The listing builds one solid part. Answer for the finished solid, in the listing's coordinates (mm). A direction names the side the tool comes from. Round coordinates to 2 decimals unless told otherwise and drop trailing zeros. Write each loop counter-clockwise with the first axis right and the second up, starting at its lowest first coordinate (ties: lowest second). Pieces come first, ordered by that corner, then holes.
from build123d import *

# Parameters (mm, degrees)
F1_DEPTH  = 210
F2_DEPTH  = 210
F3_DEPTH  = 60
F5_D      = 15
F5_DEPTH  = 40
F5_TIP    = 4.5064546427
F7_DEPTH  = 20
F9_DEPTH  = 20
F10_W     = 10
F10_H     = 20
F11_DEPTH = 210
F12_D     = 10
F12_DEPTH = 40
F12_TIP   = 3.0043030951
F13_R     = 7
F14_DEPTH = 50
F15_R     = 7
F16_DEPTH = 50
F18_D     = 15
F18_DEPTH = 220
F18_TIP   = 4.5064546427
F19_W     = 60
F19_H     = 50
F20_DEPTH = 60
F21_W     = 9.6634474397
F21_H     = 30
F21_W_2   = 10
F22_DEPTH = 20
F23_DEPTH = 25
F24_DEPTH = 31
F25_DEPTH = 37
F26_DEPTH = 45
F27_DEPTH = 120
F28_DEPTH = 105
F29_DEPTH = 200


with BuildPart() as f1:
    # F0 (on Front) → F1 (new body)
    with BuildSketch(Plane.XZ):
        with BuildLine():
            Line((-190, 0), (-210, 0))
            ThreePointArc((-210, 0), (-148.4924240492, -148.4924240492), (0, -210))
            Line((0, -210), (0, -190))
            ThreePointArc((0, -190), (-134.3502884254, -134.3502884254), (-190, 0))
        make_face()
    extrude(amount=F1_DEPTH)

    # F2 (add): a face of the model
    f2_faces = [f1.faces().sort_by_distance(p)[0] for p in [
        (-200, -105, 0),
    ]]
    extrude(f2_faces, amount=-F2_DEPTH)

    # F3 (add): a face of the model
    f3_faces = [f1.faces().sort_by_distance(p)[0] for p in [
        (0, -105, -200),
    ]]
    extrude(f3_faces, amount=-F3_DEPTH)

    # F5
    with Locations(Plane(origin=(0, 0, -210), x_dir=(1, 0, 0), z_dir=(0, 0, -1))):
        with Locations((-30, 157.5), (-30, 52.5)):
            Hole(F5_D / 2, depth=F5_DEPTH)
            with Locations((0, 0, -(F5_DEPTH + F5_TIP / 2))):  # 118° drill point
                Cone(0, F5_D / 2, F5_TIP, mode=Mode.SUBTRACT)

    # F6 (on face) → F7 (join)
    with BuildSketch(Plane.XZ.offset(210)):
        with BuildLine():
            ThreePointArc((0, -170), (-120.2081528017, -120.2081528017), (-170, 0))
            Line((-170, 0), (-190, 0))
            ThreePointArc((-190, 0), (-134.3502884254, -134.3502884254), (0, -190))
            Line((0, -190), (0, -170))
        make_face()
    extrude(amount=-F7_DEPTH)

    # F8 (on face) → F9 (join)
    with BuildSketch(Plane(origin=(0, 0, 0), x_dir=(-1, 0, 0), z_dir=(0, 1, 0))):
        with BuildLine():
            Line((190, 0), (170, 0))
            ThreePointArc((170, 0), (120.2081528017, -120.2081528017), (0, -170))
            Line((0, -170), (0, -190))
            ThreePointArc((0, -190), (134.3502884254, -134.3502884254), (190, 0))
        make_face()
    extrude(amount=-F9_DEPTH)

    # F10 (on face) → F11 (join)
    with BuildSketch(Plane.XZ.offset(210)):
        with Locations((-35, -200)):
            Rectangle(F10_W, F10_H)
        with Locations((-25, -200)):
            Rectangle(F10_W, F10_H)
    extrude(amount=-F11_DEPTH)

    # F12
    with Locations(Plane(origin=(0, 0, -210), x_dir=(1, 0, 0), z_dir=(0, 0, -1))):
        with Locations((-30, 157.5), (-30, 52.5)):
            Hole(F12_D / 2, depth=F12_DEPTH)
            with Locations((0, 0, -(F12_DEPTH + F12_TIP / 2))):  # 118° drill point
                Cone(0, F12_D / 2, F12_TIP, mode=Mode.SUBTRACT)

    # F13 (on face) → F14 (cut)
    with BuildSketch(Plane.YZ):
        with Locations((-140, -200)):
            Circle(F13_R)
        with Locations((-105, -200)):
            Circle(F13_R)
        with Locations((-70, -200)):
            Circle(F13_R)
    extrude(amount=-F14_DEPTH, mode=Mode.SUBTRACT)

    # F15 (on face) → F16 (cut)
    with BuildSketch(Plane.XY):
        with Locations((-200, -35)):
            Circle(F15_R)
        with Locations((-200, -70)):
            Circle(F15_R)
        with Locations((-200, -105)):
            Circle(F15_R)
        with Locations((-200, -140)):
            Circle(F15_R)
        with Locations((-200, -175)):
            Circle(F15_R)
    extrude(amount=-F16_DEPTH, mode=Mode.SUBTRACT)

    # F18
    with Locations(Plane.XZ.offset(210)):
        with Locations((-183.5259069949, -49.1756185695), (-164.544826719, -95), (-134.3502884254, -134.3502884254), (-49.1756185695, -183.5259069949)):
            Hole(F18_D / 2, depth=F18_DEPTH)
            with Locations((0, 0, -(F18_DEPTH + F18_TIP / 2))):  # 118° drill point
                Cone(0, F18_D / 2, F18_TIP, mode=Mode.SUBTRACT)

    # F19 (on face) → F20 (cut)
    with BuildSketch(Plane(origin=(0, 0, -210), x_dir=(1, 0, 0), z_dir=(0, 0, -1))):
        with Locations((-100, 105)):
            Rectangle(F19_W, F19_H)
    extrude(amount=-F20_DEPTH, mode=Mode.SUBTRACT)

    # F21 (on face) → F22 (join)
    with BuildSketch(Plane(origin=(0, 0, -210), x_dir=(1, 0, 0), z_dir=(0, 0, -1))):
        with Locations((-65.1682762802, 45)):
            Rectangle(F21_W, F21_H)
        with Locations((-75, 165)):
            Rectangle(F21_W_2, F21_H)
        with Locations((-65.1682762802, 165)):
            Rectangle(F21_W, F21_H)
        with Locations((-75, 45)):
            Rectangle(F21_W_2, F21_H)
        with Locations((-85, 165)):
            Rectangle(F21_W_2, F21_H)
        with Locations((-85, 45)):
            Rectangle(F21_W_2, F21_H)
    extrude(amount=-F22_DEPTH)

    # F21 (on face) → F23 (join)
    with BuildSketch(Plane(origin=(0, 0, -210), x_dir=(1, 0, 0), z_dir=(0, 0, -1))):
        with Locations((-95, 165)):
            Rectangle(F21_W_2, F21_H)
        with Locations((-95, 45)):
            Rectangle(F21_W_2, F21_H)
    extrude(amount=-F23_DEPTH)

    # F21 (on face) → F24 (join)
    with BuildSketch(Plane(origin=(0, 0, -210), x_dir=(1, 0, 0), z_dir=(0, 0, -1))):
        with Locations((-105, 165)):
            Rectangle(F21_W_2, F21_H)
        with Locations((-105, 45)):
            Rectangle(F21_W_2, F21_H)
    extrude(amount=-F24_DEPTH)

    # F21 (on face) → F25 (join)
    with BuildSketch(Plane(origin=(0, 0, -210), x_dir=(1, 0, 0), z_dir=(0, 0, -1))):
        with Locations((-115, 165)):
            Rectangle(F21_W_2, F21_H)
        with Locations((-115, 45)):
            Rectangle(F21_W_2, F21_H)
    extrude(amount=-F25_DEPTH)

    # F21 (on face) → F26 (join)
    with BuildSketch(Plane(origin=(0, 0, -210), x_dir=(1, 0, 0), z_dir=(0, 0, -1))):
        with Locations((-125, 45)):
            Rectangle(F21_W_2, F21_H)
        with Locations((-125, 165)):
            Rectangle(F21_W_2, F21_H)
    extrude(amount=-F26_DEPTH)

    # F21 (on face) → F27 (join)
    with BuildSketch(Plane(origin=(0, 0, -210), x_dir=(1, 0, 0), z_dir=(0, 0, -1))):
        with Locations((-185, 165)):
            Rectangle(F21_W_2, F21_H)
        with Locations((-185, 45)):
            Rectangle(F21_W_2, F21_H)
    extrude(amount=-F27_DEPTH)

    # F21 (on face) → F28 (join)
    with BuildSketch(Plane(origin=(0, 0, -210), x_dir=(1, 0, 0), z_dir=(0, 0, -1))):
        with Locations((-175, 165)):
            Rectangle(F21_W_2, F21_H)
        with Locations((-175, 45)):
            Rectangle(F21_W_2, F21_H)
    extrude(amount=-F28_DEPTH)

    # F13 (on face) → F29 (cut)
    with BuildSketch(Plane.YZ):
        with Locations((-35, -200)):
            Circle(F13_R)
        with Locations((-175, -200)):
            Circle(F13_R)
    extrude(amount=-F29_DEPTH, mode=Mode.SUBTRACT)


solid = f1.part
1. Straight lines are drawn through the part: line 1 along Y through (x, z) = (-30, -188); line 2 along Y through (x, z) = (-188, -16.5); line 3 along X through (y, z) = (-52.5, -194.5). For each, find the intervals that lie inside material, in ascending order.
Geometry says:
line 1: y = -210 to -165, -150 to -60, -45 to 0
line 2: y = -210 to -190, -20 to 0
line 3: x = -210 to -170, -130 to -35, -25 to 0
2. Section A-A on z = -95 is taken. Determine the outline of the cut face in (x, y).
Geometry says:
outline: (-210, -210) - (-190, -210) - (-190, -180) - (-187.28, -180) - (-187.28, -210) - (-172.04, -210) - (-172.04, 0) - (-187.28, 0) - (-187.28, -30) - (-190, -30) - (-190, 0) - (-210, 0) - close; (-157.04, -210) - (-140.98, -210) - (-140.98, -190) - (-157.04, -190) - close; (-157.04, -20) - (-140.98, -20) - (-140.98, 0) - (-157.04, 0) - close; hole (-190, -150) - (-187.28, -150) - (-187.28, -60) - (-190, -60) - close
3. A tool of negligible diameter and unlimited length cuts with its end or side. For faces 5 (the face through (-50, -140, -200)), 6 (the face through (-103, -150, -198)), 7 (the face through (-193.323, -102.897, -24.65)), 8 (the face through (-20.78, -103.81, -188.86)), from which of +Z, -Z, +X, -X, +Y, -Y can it reach the whole face along a straight path? Write none if from no direction.
Geometry says:
face 5: +X
face 6: -Z
face 7: +Z
face 8: +Z, +X
4. Section C-C on x = -146 is taken. Determine the outline of the cut face in (y, z).
Geometry says:
outline: (-210, -150.94) - (0, -150.94) - (0, -87.09) - (-20, -87.09) - (-20, -121.59) - (-190, -121.59) - (-190, -87.09) - (-210, -87.09) - close
5. Given pin 1 (6 mm diameter, centred on x = -136, y = -136, fed in from +Z) (3 decimals); pin 2 (4 mm diameter, centred on x = -200.5, y = -68, fed in from +Z); pin 3 (5.5 mm diameter, centred on x = -100, z = -207.5, fed in from -Y), each flat-ended and moving along its own axis, determine where each tip first touches the part or whether it passes through.
Geometry says:
pin 1: stops at z = -140.235
pin 2: stops at z = -50
pin 3: stops at y = -180
6. For a pull along Y with two mould halves and no side action, classify faces 1 (the face through (-35, -51, -190)), 2 (the face through (-144, -210, -128)), 3 (the face through (-116, -30, -187)), 4 (the face through (-118.9, -200.1, -121.5)) as released by +Y, released by -Y, zero draft, split by the parting line, or undercut.
Geometry says:
face 1: undercut
face 2: released by -Y
face 3: released by +Y
face 4: zero draft
7. Section B-B on y = -140 is taken. Determine the outline of the cut face in (x, z).
Geometry says:
outline: (-210, -210) - (-190, -210) - (-190, -89.44) arc R210 ccw to (-60, -201.25) - (-60, -210) - (0, -210) - (0, -207) - (-50, -207) - (-50, -193) - (0, -193) - (0, -190) arc R190 cw to (-41.89, -185.32) arc R7.5 cw (long way) to (-56.38, -181.44) arc R190 cw to (-128.94, -139.55) arc R7.5 cw (long way) to (-139.55, -128.94) arc R190 cw to (-160.67, -101.42) arc R7.5 cw (long way) to (-168.17, -88.43) arc R190 cw to (-181.44, -56.38) arc R7.5 cw (long way) to (-185.32, -41.89) arc R190 cw to (-190, 0) - (-193, 0) - (-193, -50) - (-207, -50) - (-207, 0) - (-210, 0) - close
